For this review, use the dimensioned drawing (mm, ordinates from the lowest corner) and the shaded views. A direction names the side the tool comes from. Coordinates: 2 decimals unless noted, no trailing zeros. Write each loop counter-clockwise with the first axis right and the second up, starting at its lowest first coordinate (ties: lowest second). Pieces come first, ordered by that corner, then holes. Notation, with made-up numbers: (-38.5, 19) - (-12.5, 19) arc R22 cw to (-12.5, 27) - close; hole circle Ø2 at (41.5, -25). An arc over 180 degrees is marked (long way). One line per item, written item: value.
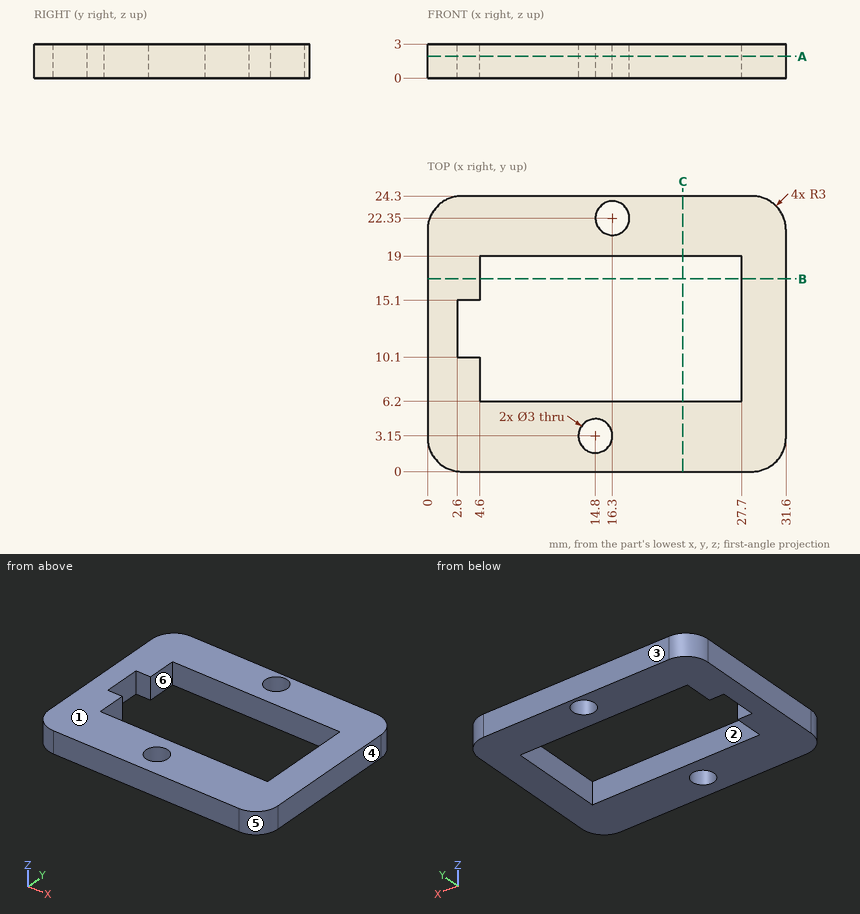
1. Wall thickness on line 1 along Y through (x, z) = (11.5, 2.7); line 2 along X through (y, z) = (10.75, 1.7); line 3 along X through (y, z) = (2.25, 2): over which ranges is each line inside the solid? List them lowest first.
Answer block:
line 1: y = 0 to 6.2, 19 to 24.3
line 2: x = 0 to 2.6, 27.7 to 31.6
line 3: x = 0.1 to 13.6, 16 to 31.5
2. Consider section B-B, the plane y = 17. Write out the cut boundary in (x, z).
Answer block:
outline: (0, 0) - (4.6, 0) - (4.6, 3) - (0, 3) - close; (27.7, 0) - (31.6, 0) - (31.6, 3) - (27.7, 3) - close
3. Consider section A-A, the plane z = 1.9. Write out the cut boundary in (x, y).
Answer block:
outline: (0, 3) arc R3 ccw to (3, 0) - (28.6, 0) arc R3 ccw to (31.6, 3) - (31.6, 21.3) arc R3 ccw to (28.6, 24.3) - (3, 24.3) arc R3 ccw to (0, 21.3) - close; hole (2.6, 10.1) - (4.6, 10.1) - (4.6, 6.2) - (27.7, 6.2) - (27.7, 19) - (4.6, 19) - (4.6, 15.1) - (2.6, 15.1) - close; hole circle Ø3 at (14.8, 3.15); hole circle Ø3 at (16.3, 22.35)
4. Insertion check: pin 1 Ø4 at (x, y) = (26, 13) entering from +Z. The pin has a flat end and moves straight along its axis. Give the tip position at first contact, or say it passes through.
Answer block:
pin 1: stops at z = 3
5. Mouldability with a two-part tool opening along Y and no side actions: class the marked faces 3, 4, 5 and 6 as released by +Y, released by -Y, zero draft, split by the parting line, or undercut.
Answer block:
face 3: released by +Y
face 4: zero draft
face 5: released by -Y
face 6: undercut
6. Consider section C-C, the plane x = 22.5. Write out the cut boundary in (y, z).
Answer block:
outline: (0, 0) - (6.2, 0) - (6.2, 3) - (0, 3) - close; (19, 0) - (24.3, 0) - (24.3, 3) - (19, 3) - close
7. For the marked faces 1 and 2, list the 3-axis set-ups (+Z, -Z, +X, -X, +Y, -Y) from which the entire face can be reached by the end or side of a thin tool; tool diameter is ignored.
Answer block:
face 1: +Z, +X, -X, +Y, -Y
face 2: +Z, -Z
